Read the model definition and answer for the solid it produces. Units are mm, in the model's axes. Face numbers are marked on the shaded views. Round coordinates to 2 decimals unless told otherwise and drop trailing zeros. Write each loop counter-clockwise with the first axis right and the second up, starting at its lowest first coordinate (ties: lowest second). Pieces come first, ordered by that corner, then holes. Notation, with made-up numbers: M 40.5,80 L 63.5,80 A20 ccw 63.5,111 Z; hole C -24.5,-25 d4. An arc over 180 degrees is marked long. Use one line per item in the form item = value. Start each with the question number.
```python
from build123d import *

# Parameters (mm, degrees)
F1_DEPTH = 3.5
F2_W     = 38.9
F2_H     = 8.6
F3_DEPTH = 2.5


with BuildPart() as f1:
    # F0 (on Top) → F1 (new body)
    with BuildSketch(Plane.XY):
        with BuildLine():
            Line((-17.5, -12), (17.5, -12))
            ThreePointArc((17.5, -12), (20.328427, -10.828427), (21.5, -8))
            Line((21.5, -8), (21.5, 8))
            ThreePointArc((21.5, 8), (20.328427, 10.828427), (17.5, 12))
            Line((17.5, 12), (-17.5, 12))
            ThreePointArc((-17.5, 12), (-20.328427, 10.828427), (-21.5, 8))
            Line((-21.5, 8), (-21.5, -8))
            ThreePointArc((-21.5, -8), (-20.328427, -10.828427), (-17.5, -12))
        make_face()
    extrude(amount=F1_DEPTH)

    # F2 (on face) → F3 (cut)
    with BuildSketch(Plane.XY.offset(3.5)):
        with Locations((0, 5.113459)):
            Rectangle(F2_W, F2_H)
    extrude(amount=-F3_DEPTH, mode=Mode.SUBTRACT)


solid = f1.part
```
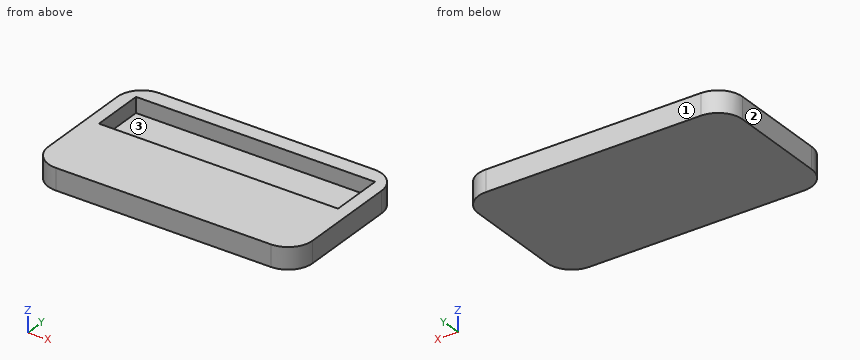
Q1. Find section C-C on x = 7. Write down the section's boundary in (y, z), and give its area (3 significant figures).
Q2. This flat-tipped pin is pushed along its axis until it touches: pin 1 Ø4.5 at (x, y) = (7, 4) entering from +Z. Where does it stop, or does it pass through?
Q3. Find section D-D on y = -10. Write down the section's boundary in (x, z).
Q4. Find section A-A on y = 4.5. Write down the section's boundary in (x, z).
Q5. For a pull along X with two mould halves and no side action, classify the marked faces 1, 2 and 3 as +X half, -X half, draft (parallel to the pull), parting line (faces both ways), or undercut.
Q6. Straight lines are drawn through the part: line 1 (Y direction, x = 12, z = 2.95); line 2 (X direction, y = 4, z = 2.5); line 3 (Z direction, x = 2, y = 6). For each, find the intervals that lie inside material, in ascending order. Write a range as [from, to].
Q7. Find section B-B on z = 2.2. Write down the section's boundary in (x, y).
Response:
q1.outline = M -12,0 L 12,0 L 12,3.5 L 9.41,3.5 L 9.41,1 L 0.81,1 L 0.81,3.5 L -12,3.5 Z
q1.area = 62.5 mm²
q2.pin_1 = 1
q3.outline = M -20.96,0 L 20.96,0 L 20.96,3.5 L -20.96,3.5 Z
q4.outline = M -21.5,0 L 21.5,0 L 21.5,3.5 L 19.45,3.5 L 19.45,1 L -19.45,1 L -19.45,3.5 L -21.5,3.5 Z
q5.face_1 = draft
q5.face_2 = -X half
q5.face_3 = undercut
q6.line_1 = [-12, 0.81], [9.41, 12]
q6.line_2 = [-21.5, -19.45], [19.45, 21.5]
q6.line_3 = [0, 1]
q7.outline = M -21.5,-8 A4 ccw -17.5,-12 L 17.5,-12 A4 ccw 21.5,-8 L 21.5,8 A4 ccw 17.5,12 L -17.5,12 A4 ccw -21.5,8 Z; hole M -19.45,0.81 L 19.45,0.81 L 19.45,9.41 L -19.45,9.41 Z
